Build history of the part. All positions in model axes, mm. Face numbers are marked on the shaded views. A direction names the side the tool comes from. Round coordinates to 2 decimals unless told otherwise and drop trailing zeros. Write each loop counter-clockwise with the first axis right and the second up, starting at its lowest first coordinate (ties: lowest second). Pieces come first, ordered by that corner, then holes. Notation, with made-up numbers: (27.5, -33) -> (66.5, -33) arc R13 cw to (66.5, -16) -> close; hole circle Ø3 at (30.5, 30.25). An arc over 180 degrees is marked (long way). Answer in a Markdown table with one row per item.
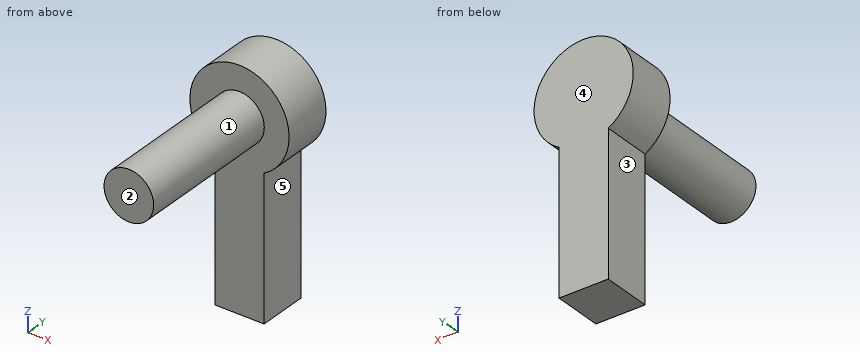
```python
from build123d import *

# Parameters (mm, degrees)
SKETCH1_R           = 3.175
BOSS_EXTRUDE1_DEPTH = 19.05
BOSS_EXTRUDE2_DEPTH = 6.35
SKETCH4_W           = 6.30056433
SKETCH4_H           = 6.35
BOSS_EXTRUDE3_DEPTH = 14.986


with BuildPart() as part:
    # Sketch1 → Boss-Extrude1 (new body)
    with BuildSketch(Plane(origin=(0, 0, 0), x_dir=(1, 0, 0), z_dir=(0, 1, 0))):
        Circle(SKETCH1_R)
    extrude(amount=BOSS_EXTRUDE1_DEPTH)

    # Sketch3 → Boss-Extrude2 (add)
    with BuildSketch(Plane(origin=(0, 19.05, 0), x_dir=(1, 0, 0), z_dir=(0, 1, 0))):
        with BuildLine():
            Line((3.150282165, 5.513458287), (3.150282165, 8.686029988))
            Line((3.150282165, 8.686029988), (-3.150282165, 8.686029988))
            Line((-3.150282165, 8.686029988), (-3.150282165, 5.513458287))
            ThreePointArc((-3.150282165, 5.513458287), (0, -6.35), (3.150282165, 5.513458287))
        make_face()
    extrude(amount=BOSS_EXTRUDE2_DEPTH)

    # Sketch4 → Boss-Extrude3 (add)
    with BuildSketch(Plane(origin=(0, 0, -8.686029988), x_dir=(-1, 0, 0), z_dir=(0, 0, -1))):
        with Locations((0, 22.225)):
            Rectangle(SKETCH4_W, SKETCH4_H)
    extrude(amount=BOSS_EXTRUDE3_DEPTH)


solid = part.part
```
Q1. Which spindle directions (+Z, -Z, +X, -X, +Y, -Y) get a long thin tool onto all of the face, cutting with end or side? Do the marked faces 1, 2, 3, 4 and 5. Say none if no direction does.
A:
| item | result |
|---|---|
| face 1 | -Y |
| face 2 | +Z, -Z, +X, -X, -Y |
| face 3 | -Z, -X, +Y, -Y |
| face 4 | +Z, -Z, +X, -X, +Y |
| face 5 | -Z, +X, +Y, -Y |
Q2. Saw through at B-B on z = 0. Write the cut outline in (x, y) (3 decimals), plus the area to 3 significant figures.
A:
| item | result |
|---|---|
| outline | (-6.35, 19.05) -> (-3.175, 19.05) -> (-3.175, 0) -> (3.175, 0) -> (3.175, 19.05) -> (6.35, 19.05) -> (6.35, 25.4) -> (-6.35, 25.4) -> close |
| area | 202 mm² |
Q3. Saw through at C-C on y = 15.5. Write the cut outline in (x, z) (3 decimals).
A:
| item | result |
|---|---|
| outline | circle Ø6.35 at (0, 0) |
Q4. Drop flat-ended pins along their axis: P1, Ø3, axis at y = 21.5, z = -15.5, coming from the +X side; P2, Ø4, axis at x = -2.5, y = 22.5, coming from the +Z side; P3, Ø4, axis at x = 2.5, z = -15, coming from the -Y side. Give the stop position or say it passes through.
A:
| item | result |
|---|---|
| P1 | x = 3.15 |
| P2 | z = 6.33 |
| P3 | y = 19.05 |
Q5. Saw through at D-D on z = -15.5. Write the cut outline in (x, y).
A:
| item | result |
|---|---|
| outline | (-3.15, 19.05) -> (3.15, 19.05) -> (3.15, 25.4) -> (-3.15, 25.4) -> close |
Q6. Saw through at A-A on x = 0. Write the cut outline in (y, z) (3 decimals), plus the area to 3 significant figures.
A:
| item | result |
|---|---|
| outline | (0, -3.175) -> (19.05, -3.175) -> (19.05, -23.672) -> (25.4, -23.672) -> (25.4, 6.35) -> (19.05, 6.35) -> (19.05, 3.175) -> (0, 3.175) -> close |
| area | 312 mm² |
Q7. Wall check: line 1 (X direction, y = 21, z = -21); line 2 (Y direction, x = 1, z = -14.5); line 3 (Z direction, x = -0.5, y = 12.25). Give the ranges that are in metal, low to high. Write a range as [from, to].
A:
| item | result |
|---|---|
| line 1 | [-3.15, 3.15] |
| line 2 | [19.05, 25.4] |
| line 3 | [-3.14, 3.14] |
